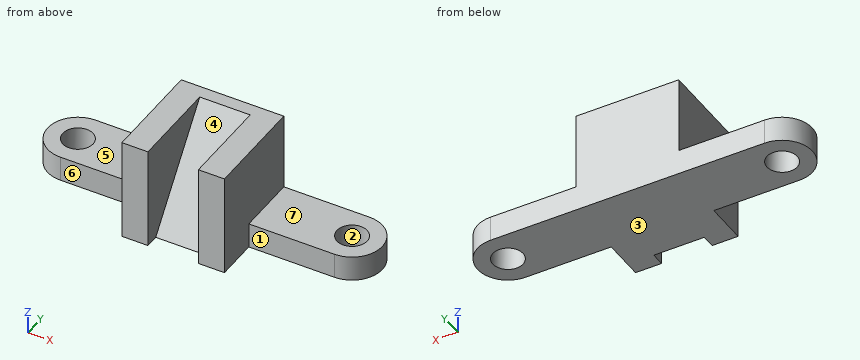
```python
from build123d import *

# Parameters (mm, degrees)
F1_DEPTH = 61
F3_DEPTH = 30
F0_R     = 9
F4_DEPTH = 15


with BuildPart() as f1:
    # F0 (on Top) → F1 (new body)
    with BuildSketch(Plane.XY):
        Polygon((-2.163718, 11.050885), (-2.163718, -13.949115), (13.336282, -13.949115), (13.336282, 39.300885), (43.336282, 39.300885), (43.336282, -13.949115), (58.836282, -13.949115), (58.836282, 11.050885), (58.836282, 47.050885), (-2.163718, 47.050885), align=None)
    extrude(amount=F1_DEPTH)

    # F2 (on face) → F3 (join)
    with BuildSketch(Plane(origin=(43.336282, 0, 0), x_dir=(0, -1, 0), z_dir=(-1, 0, 0))):
        Polygon((-39.300885, 0), (5.949115, 0), (-39.300885, 61), align=None)
    extrude(amount=F3_DEPTH)

    # F0 (on Top) → F4 (join)
    with BuildSketch(Plane.XY):
        with BuildLine():
            Line((-53.163718, 11.050885), (-2.163718, 11.050885))
            Line((-2.163718, 11.050885), (-2.163718, 47.050885))
            Line((-2.163718, 47.050885), (-53.163718, 47.050885))
            ThreePointArc((-53.163718, 47.050885), (-71.163718, 29.050885), (-53.163718, 11.050885))
        make_face()
        with Locations((-53.163718, 29.050885)):
            Circle(F0_R, mode=Mode.SUBTRACT)
        with BuildLine():
            Line((109.836282, 47.050885), (58.836282, 47.050885))
            Line((58.836282, 47.050885), (58.836282, 11.050885))
            Line((58.836282, 11.050885), (109.836282, 11.050885))
            ThreePointArc((109.836282, 11.050885), (127.836282, 29.050885), (109.836282, 47.050885))
        make_face()
        with Locations((109.836282, 29.050885)):
            Circle(F0_R, mode=Mode.SUBTRACT)
    extrude(amount=F4_DEPTH)


solid = f1.part
```
Source: CAD feature listing. Evaluate the final solid. Frame: model axes, mm. Face numbers are marked on the shaded views. A direction names the side the tool comes from. Round coordinates to 2 decimals unless told otherwise and drop trailing zeros. Write each loop counter-clockwise with the first axis right and the second up, starting at its lowest first coordinate (ties: lowest second). Pieces come first, ordered by that corner, then holes. Notation, with made-up numbers: M -9.5,9.5 L 1.5,9.5 A31 cw 1.5,45.5 Z; hole C -22.75,-32.5 d3. An arc over 180 degrees is marked long. Answer as a JSON object with one key per item and string values. Group by question number.
(1) Reachability of the marked faces 4, 5, 6 and 7 from +Z, -Z, +X, -X, +Y, -Y: full face, straight path, thin tool, end or side. Return the list, or none.
(2) Mould query, pull axis Y, two halves, no side actions, for the marked faces 1, 2 and 3. Classes: +Y half, -Y half, draft (parallel to the pull), parting line (faces both ways), or undercut.
(3) Section query B-B on z = 10. Output: boundary loops of the cut face in (x, y).
(4) First-contact query: pin 1 (3 mm diameter, centred on y = 24.5, z = 17.5, fed in from -X); pin 2 (18 mm diameter, centred on x = -32, y = 33, fed in from +Z); pin 3 (2 mm diameter, centred on y = -6, z = 42.5, fed in from +X). Flat tips, straight axial feed; report the tip coordinate or a pass-through.
(5) Section query D-D on y = 18. Output: boundary loops of the cut face in (x, z) (3 decimals), then the cut area to 3 significant figures.
(6) Section query C-C on z = 51.5. Output: boundary loops of the cut face in (x, y), then the cut area to 3 significant figures.
(7) Ray query, line 1 (X direction, y = -3, z = 21); line 2 (X direction, y = 25, z = 30.5); line 3 (Z direction, x = -16, y = 16.5). Return the intervals inside material, ascending. Write a range as [from, to].
(8) Section query A-A on x = 113. Output: boundary loops of the cut face in (y, z), then the cut area to 3 significant figures.
Computed values:
{
 "1": {"face 4": "+Z, -Y", "face 5": "+Z, -X, +Y, -Y", "face 6": "+Z, -Z, -X, -Y", "face 7": "+Z, +X, +Y, -Y"},
 "2": {"face 1": "-Y half", "face 2": "undercut", "face 3": "draft"},
 "3": {"outline": "M -53.16,11.05 L -2.16,11.05 L -2.16,-13.95 L 13.34,-13.95 L 13.34,1.47 L 43.34,1.47 L 43.34,-13.95 L 58.84,-13.95 L 58.84,11.05 L 109.84,11.05 A18 ccw 109.84,47.05 L -53.16,47.05 A18 ccw Z; hole C -53.16,29.05 d18; hole C 109.84,29.05 d18"},
 "4": {"pin 1": "x = -2.16", "pin 2": "z = 15", "pin 3": "x = 58.84"},
 "5": {"outline": "M -67.372,0 L 124.045,0 L 124.045,15 L 58.836,15 L 58.836,61 L 43.336,61 L 43.336,32.285 L 13.336,32.285 L 13.336,61 L -2.164,61 L -2.164,15 L -67.372,15 Z", "area": "4,820 mm^2"},
 "6": {"outline": "M -2.16,-13.95 L 13.34,-13.95 L 13.34,32.25 L 43.34,32.25 L 43.34,-13.95 L 58.84,-13.95 L 58.84,47.05 L -2.16,47.05 Z", "area": "2,330 mm^2"},
 "7": {"line 1": "[-2.16, 13.34], [43.34, 58.84]", "line 2": "[-2.16, 58.84]", "line 3": "[0, 15]"},
 "8": {"outline": "M 11.33,0 L 20.63,0 L 20.63,15 L 11.33,15 Z; M 37.48,0 L 46.77,0 L 46.77,15 L 37.48,15 Z", "area": "279 mm^2"}
}
